```python
from build123d import *

# Parameters (mm, degrees)
BOSS_EXTRUDE1_DEPTH = 8
SKETCH2_R           = 6
BOSS_EXTRUDE2_DEPTH = 40
FILLET1_R           = 1


with BuildPart() as part:
    # Sketch1 → Boss-Extrude1 (new body)
    with BuildSketch(Plane(origin=(0, 0, 0), x_dir=(1, 0, 0), z_dir=(0, 1, 0))):
        Polygon((9.799334365, -3.115685798), (9.132298337, 4.726053225), (3.115685798, 9.799334365), (-4.726053225, 9.132298337), (-9.799334365, 3.115685798), (-9.132298337, -4.726053225), (-3.115685798, -9.799334365), (4.726053225, -9.132298337), align=None)
    extrude(amount=BOSS_EXTRUDE1_DEPTH)

    # Sketch2 → Boss-Extrude2 (add)
    with BuildSketch(Plane.XZ):
        with Locations(Location((0, 0, 0), (0, 0, 90))):
            Circle(SKETCH2_R)
    extrude(amount=BOSS_EXTRUDE2_DEPTH)

    # Fillet1
    fillet1_edges = [part.edges().sort_by_distance(p)[0] for p in [
        (-9.465816351, 8, 0.805183713),
        (-7.262693795, 0, -6.123992067),
        (-0.805183713, 0, -9.465816351),
        (-6.123992067, 8, 7.262693795),
        (0.805183713, 8, 9.465816351),
        (7.262693795, 8, 6.123992067),
        (9.465816351, 8, -0.805183713),
        (6.123992067, 8, -7.262693795),
        (-0.805183713, 8, -9.465816351),
        (-7.262693795, 8, -6.123992067),
        (6.123992067, 0, -7.262693795),
        (9.465816351, 0, -0.805183713),
        (7.262693795, 0, 6.123992067),
        (0.805183713, 0, 9.465816351),
        (-6.123992067, 0, 7.262693795),
        (-9.465816351, 0, 0.805183713),
    ]]
    fillet(fillet1_edges, radius=FILLET1_R)


solid = part.part
```
Check sheet for the modelled part. Datum: model origin and axes. Units: mm. Round coordinates to 2 decimals unless told otherwise and drop trailing zeros. Order: outer loops, then holes, each group sorted by start corner. A loop starts at its lowest first (then second) coordinate and runs counter-clockwise, first axis right, second up.
1) Section check B-B (y = -22). Record the boundary of the cut face in (x, z).
2) Scan lines: line 1 (Y direction, x = -4.25, z = -7); line 2 (X direction, y = -37, z = 2); line 3 (Y direction, x = -4.5, z = 8). Record each from-to range of solid material in increasing order.
3) Go/stop test with flat-tipped pins: pin 1 Ø5 at (x, y) = (-6, 1.5) entering from +Z; pin 2 Ø8 at (y, z) = (-33, -3) entering from -X; pin 3 Ø2 at (x, z) = (4, -6.5) entering from -Y. Record where each tip stops, or that it passes through.
4) Section check A-A (y = 1.5). Record the boundary of the cut face in (x, z).
Result:
1. outline: circle Ø12 at (0, 0)
2. line 1: y = 0 to 8
2. line 2: x = -5.66 to 5.66
2. line 3: y = 0.14 to 7.86
3. pin 1: stops at z = 9.48
3. pin 2: stops at x = -6
3. pin 3: stops at y = 0
4. outline: (-9.8, -3.12) - (-4.73, -9.13) - (3.12, -9.8) - (9.13, -4.73) - (9.8, 3.12) - (4.73, 9.13) - (-3.12, 9.8) - (-9.13, 4.73) - close
